Can you work these out from the model? Positions are in its coordinate system, mm. A direction names the side the tool comes from. Give positions to 0.01 mm unless a question says otherwise; leave off trailing zeros. Order: outer loops, then holes, each group sorted by start corner. A loop starts at its lowest first (then second) coordinate and runs counter-clockwise, first axis right, second up. Notation, with made-up numbers: M 68,-26.5 L 126,-26.5 A15 ccw 126,-20.5 Z; hole C -16,-4 d3. An arc over 180 degrees is marked long. Write each question's results on one line, items separated by ' | '.
from build123d import *

# Parameters (mm, degrees)
SKETCH1_W           = 81.28
SKETCH1_H           = 62.23
BOSS_EXTRUDE1_DEPTH = 3.175
FILLET1_R           = 2.54


with BuildPart() as part:
    # Sketch1 → Boss-Extrude1 (new body)
    with BuildSketch(Plane(origin=(0, 0, 0), x_dir=(1, 0, 0), z_dir=(0, 1, 0))):
        Polygon((103.066957551, 0), (81.28, 31.115), (81.28, 0), align=None)
        with Locations((40.64, 31.115)):
            Rectangle(SKETCH1_W, SKETCH1_H)
    extrude(amount=BOSS_EXTRUDE1_DEPTH)

    # Fillet1
    fillet1_edges = [part.edges().sort_by_distance(p)[0] for p in [
        (0, 1.5875, 0),
        (81.28, 1.5875, -31.115),
        (103.066957551, 1.5875, 0),
    ]]
    fillet(fillet1_edges, radius=FILLET1_R)


solid = part.part
(1) Imagine slicing it at C-C, the plane z = -23. Write out the boundary of the cut face in (x, y) (3 decimals), plus the area to 3 significant figures.
Data:
outline: M 0,0 L 86.962,0 L 86.962,3.175 L 0,3.175 Z | area: 276 mm2
(2) Imagine slicing it at A-A, the plane y = 2.1. Write out the boundary of the cut face in (x, z).
Data:
outline: M 0,-62.23 L 81.28,-62.23 L 81.28,-31.92 A2.54 cw 81.74,-30.46 L 100.27,-4 A2.54 ccw 98.19,0 L 2.54,0 A2.54 ccw 0,-2.54 Z
(3) I need wall thicknesses on L1, parallel to X at y = 2.9, z = -60; L2, parallel to X at y = 1.4, z = -15.5; L3, parallel to Z at x = 84.5, y = 1.15. Which ranges of each line are inside material? Lowest first, please. Write a range as from..to.
Data:
L1: x = 0..81.28 | L2: x = 0..92.21 | L3: z = -26.52..0
(4) Imagine slicing it at B-B, the plane z = -40. Write out the boundary of the cut face in (x, y) (3 decimals).
Data:
outline: M 0,0 L 81.28,0 L 81.28,3.175 L 0,3.175 Z
(5) For faces 1 (the face through (0, 2, -32)), 2 (the face through (81.28, 2, -47)), which set-ups out of +Z, -Z, +X, -X, +Y, -Y let a thin tool reach every point of the face, with its end or its side?
Data:
face 1: +Z, -Z, -X, +Y, -Y | face 2: -Z, +X, +Y, -Y
